The model under review builds one solid part; all positions refer to its coordinate system, in mm. A direction names the side the tool comes from. Round coordinates to 2 decimals unless told otherwise and drop trailing zeros.
Item 1: Draft analysis for pull direction Z (two halves, no side actions). For faces 4 (the face through (-166.5, 5, 124)), 5 (the face through (-164.5, 5, 71)), 6 (the face through (71, 5, 164.5)), 7 (the face through (164.5, 5, 71)), state which applies: +Z half, -Z half, draft (parallel to the pull), parting line (faces both ways), or undercut.
Item 2: Clearance check with flat-ended pins moving along their axes: pin 1 Ø1.5 at (x, y) = (-72.5, 4) entering from -Z; pin 2 Ø4 at (x, z) = (120, -52.5) entering from -Y; pin 3 Ø3 at (y, z) = (5.5, 70) entering from -X; pin 4 Ø3 at (y, z) = (5, -69) entering from +X. State where each tip first meets the part, or that it passes through.
Item 3: Machinability: for faces 1 (the face through (164.5, 5, -71)), 2 (the face through (-164.5, 5, -71)), 3 (the face through (71, 5, -164.5)), which of the approach directions +Z, -Z, +X, -X, +Y, -Y give a long, thin tool a straight path to every point of the face, cutting with its end or side? Answer none if there is none.
Item 4: To check wall thickness, follow L1, parallel to X at y = 6, z = 75.5; L2, parallel to X at y = 3.75, z = -79.5. State the ranges of each line that lie inside material, in increasing order.
```python
from build123d import *

# Parameters (mm, degrees)
SKETCH1_W           = 333
SKETCH1_H           = 333
BOSS_EXTRUDE1_DEPTH = 10
CUT_EXTRUDE1_DEPTH  = 11


with BuildPart() as part:
    # Sketch1 → Boss-Extrude1 (new body)
    with BuildSketch(Plane(origin=(0, 0, 0), x_dir=(1, 0, 0), z_dir=(0, 1, 0))):
        Rectangle(SKETCH1_W, SKETCH1_H)
    extrude(amount=BOSS_EXTRUDE1_DEPTH)

    # Sketch2 → Cut-Extrude1 (cut, through all)
    with BuildSketch(Plane(origin=(0, 10, 0), x_dir=(1, 0, 0), z_dir=(0, 1, 0))):
        with BuildLine():
            Line((-77.75, -164.5), (-64.25, -164.5))
            ThreePointArc((-64.25, -164.5), (-62.835786438, -165.085786438), (-62.25, -166.5))
            Line((-62.25, -166.5), (-62.25, -168.5))
            Line((-62.25, -168.5), (-79.75, -168.5))
            Line((-79.75, -168.5), (-79.75, -166.5))
            ThreePointArc((-79.75, -166.5), (-79.164213562, -165.085786438), (-77.75, -164.5))
        make_face()
        with BuildLine():
            Line((166.5, -62.25), (168.5, -62.25))
            Line((168.5, -62.25), (168.5, -79.75))
            Line((168.5, -79.75), (166.5, -79.75))
            ThreePointArc((166.5, -79.75), (165.085786438, -79.164213562), (164.5, -77.75))
            Line((164.5, -77.75), (164.5, -64.25))
            ThreePointArc((164.5, -64.25), (165.085786438, -62.835786438), (166.5, -62.25))
        make_face()
        with BuildLine():
            Line((62.25, -166.5), (62.25, -168.5))
            Line((62.25, -168.5), (79.75, -168.5))
            Line((79.75, -168.5), (79.75, -166.5))
            ThreePointArc((79.75, -166.5), (79.164213562, -165.085786438), (77.75, -164.5))
            Line((77.75, -164.5), (64.25, -164.5))
            ThreePointArc((64.25, -164.5), (62.835786438, -165.085786438), (62.25, -166.5))
        make_face()
        with BuildLine():
            Line((168.5, 62.25), (168.5, 79.75))
            Line((168.5, 79.75), (166.5, 79.75))
            ThreePointArc((166.5, 79.75), (165.085786438, 79.164213562), (164.5, 77.75))
            Line((164.5, 77.75), (164.5, 64.25))
            ThreePointArc((164.5, 64.25), (165.085786438, 62.835786438), (166.5, 62.25))
            Line((166.5, 62.25), (168.5, 62.25))
        make_face()
        with BuildLine():
            Line((-166.5, 62.25), (-168.5, 62.25))
            Line((-168.5, 62.25), (-168.5, 79.75))
            Line((-168.5, 79.75), (-166.5, 79.75))
            ThreePointArc((-166.5, 79.75), (-165.085786438, 79.164213562), (-164.5, 77.75))
            Line((-164.5, 77.75), (-164.5, 64.25))
            ThreePointArc((-164.5, 64.25), (-165.085786438, 62.835786438), (-166.5, 62.25))
        make_face()
        with BuildLine():
            Line((-168.5, -62.25), (-168.5, -79.75))
            Line((-168.5, -79.75), (-166.5, -79.75))
            ThreePointArc((-166.5, -79.75), (-165.085786438, -79.164213562), (-164.5, -77.75))
            Line((-164.5, -77.75), (-164.5, -64.25))
            ThreePointArc((-164.5, -64.25), (-165.085786438, -62.835786438), (-166.5, -62.25))
            Line((-166.5, -62.25), (-168.5, -62.25))
        make_face()
        with BuildLine():
            Line((77.75, 164.5), (64.25, 164.5))
            ThreePointArc((64.25, 164.5), (62.835786438, 165.085786438), (62.25, 166.5))
            Line((62.25, 166.5), (62.25, 168.5))
            Line((62.25, 168.5), (79.75, 168.5))
            Line((79.75, 168.5), (79.75, 166.5))
            ThreePointArc((79.75, 166.5), (79.164213562, 165.085786438), (77.75, 164.5))
        make_face()
        with BuildLine():
            Line((-62.25, 166.5), (-62.25, 168.5))
            Line((-62.25, 168.5), (-79.75, 168.5))
            Line((-79.75, 168.5), (-79.75, 166.5))
            ThreePointArc((-79.75, 166.5), (-79.164213562, 165.085786438), (-77.75, 164.5))
            Line((-77.75, 164.5), (-64.25, 164.5))
            ThreePointArc((-64.25, 164.5), (-62.835786438, 165.085786438), (-62.25, 166.5))
        make_face()
    extrude(amount=-CUT_EXTRUDE1_DEPTH, mode=Mode.SUBTRACT)


solid = part.part
```
Numbers:
1. face 4: draft
1. face 5: undercut
1. face 6: +Z half
1. face 7: undercut
2. pin 1: stops at z = -164.5
2. pin 2: stops at y = 0
2. pin 3: stops at x = -164.5
2. pin 4: stops at x = 164.5
3. face 1: +X, +Y, -Y
3. face 2: -X, +Y, -Y
3. face 3: -Z, +Y, -Y
4. L1: x = -164.5 to 164.5
4. L2: x = -165.53 to 165.53
